Autodesk Inventor part; units mm, degrees
ref_plane "YZ Plane" through (0, 0, 0) normal (1, 0, 0) x (0, 1, 0)
ref_plane "XZ Plane" through (0, 0, 0) normal (0, 1, 0) x (-1, 0, 0)
ref_plane "XY Plane" through (0, 0, 0) normal (0, 0, 1) x (1, 0, 0)
sketch "Sketch1" plane through (0, 0, 0) normal (0, 0, 1) x (1, 0, 0)
  line L0 (0, 0) -> (0, 0.5)
  line L1 (0, 0.5) -> (-230, 2.5909)
  line L2 (-230, 2.5909) -> (-230, 0)
  line L3 (-230, 0) -> (0, 0)
  line L4 (-55, 0) -> (-55, 1)
  dimension "d0" = 55
  dimension "d1" = 1
  dimension "d2" = 0.5
  dimension "d10" = 230
extrude "Extrusion1" add sketch "Sketch1" along normal blind 35
sketch "Sketch2" plane through (-230, 0, 0) normal (0, -1, 0) x (1, 0, 0)
  line L0 (230, 0) -> (230, 35)
  line L1 (230, 17.5) -> (30, 17.5) construction
  line L2 (230, 12.3) -> (30, 12.3)
  line L3 (30, 22.7) -> (230, 22.7)
  arc A0 (230, 12.3) -> (230, 22.7) centre (230, 17.5) ccw
  arc A1 (30, 22.7) -> (30, 12.3) centre (30, 17.5) ccw
  point P0 (130, 17.5)
  dimension "d6" = 200
  dimension "d7" = 5.2
extrude "Extrusion2" cut sketch "Sketch2" against normal through all contours L2 A1 L3 L0
properties part number "WinderSpoolRemovalAid"
Check sheet for the modelled part. Datum: model origin and axes. Units: mm. Round coordinates to 2 decimals unless told otherwise and drop trailing zeros. Loops run counter-clockwise (first coordinate to the right, second up) from the corner with the lowest first, then second, coordinate; pieces in that order, holes last. Notation, with made-up numbers: (75.25, 33.5) - (107.25, 33.5) arc R22 cw to (107.25, 58.5) - close; hole circle Ø1 at (-11, -31). An arc over 180 degrees is marked (long way). Write item = value, one per line. Start each with the question number.
Q1. Release check for a two-part mould opening along Z. For faces 1 (the face through (-117, 0, 9)), 2 (the face through (-205.2, 1.2, 17.6)) record: pulls with the +Z half, pulls with the -Z half, needs draft (parallel to the pull), parting line crosses it, or undercut.
Q2. Section check D-D (x = -79). Record the boundary of the cut face in (y, z), plus the area to 3 significant figures.
Q3. Section check C-C (z = 4). Record the boundary of the cut face in (x, y).
Q4. Section check B-B (y = 1.6). Record the boundary of the cut face in (x, z).
Q5. Section check A-A (x = -40). Record the boundary of the cut face in (y, z), plus the area to 3 significant figures.
Q6. Thickness scan on L1, parallel to Z at x = -116, y = 0.35; L2, parallel to Y at x = -208, z = 30; L3, parallel to Y at x = -127, z = 27. Record the ranges inside material, lowest first.
Derived:
q1.face_1 = needs draft
q1.face_2 = undercut
q2.outline = (0, 0) - (1.22, 0) - (1.22, 12.3) - (0, 12.3) - close; (0, 22.7) - (1.22, 22.7) - (1.22, 35) - (0, 35) - close
q2.area = 30.0 mm^2
q3.outline = (-230, 0) - (0, 0) - (0, 0.5) - (-230, 2.59) - close
q4.outline = (-230, 0) - (-121, 0) - (-121, 12.3) - (-200, 12.3) arc R5.2 cw to (-200, 22.7) - (-121, 22.7) - (-121, 35) - (-230, 35) - close
q5.outline = (0, 0) - (0.86, 0) - (0.86, 12.3) - (0, 12.3) - close; (0, 22.7) - (0.86, 22.7) - (0.86, 35) - (0, 35) - close
q5.area = 21.2 mm^2
q6.L1 = 0 to 12.3, 22.7 to 35
q6.L2 = 0 to 2.39
q6.L3 = 0 to 1.65
